Autodesk Inventor part; units mm, degrees
ref_plane "Work Plane1" through (0, 0, 0) normal (1, 0, 0) x (0, 0, -1)
ref_plane "Work Plane2" through (-0.85, -1.65, 0) normal (0, 0, 1) x (1, 0, 0)
ref_plane "Work Plane3" through (-0.85, -1.65, 0) normal (0, 0, 1) x (1, 0, 0)
ref_plane "Work Plane1" through (0, 0, 0) normal (1, 0, 0) x (0, 0, -1)
sketch "Sketch3" plane through (0, 0, 0) normal (1, 0, 0) x (0, 0, -1)
  circle A0 centre (-2.6765, 0) radius 4.3638
  line L0 (-7.0404, 0) -> (1.6873, 0)
  line L1 (-0.0184, 0) -> (-0.0184, 3.4608)
  point P0 (0, 0)
ref_plane "Work Plane2" through (-0.85, -1.65, 0) normal (0, 0, 1) x (1, 0, 0)
sketch "Sketch5" plane through (-0.85, -1.65, 0) normal (0, 0, 1) x (1, 0, 0)
  line L0 (-0.8, 2.5) -> (0, 3.3)
  line L1 (-0.8, 0.8) -> (-0.8, 2.5)
  line L2 (0, 0) -> (-0.8, 0.8)
  line L3 (2.5, 0) -> (0, 0)
  line L4 (2.5, 3.3) -> (2.5, 0)
  line L5 (0, 3.3) -> (2.5, 3.3)
  circle A0 centre (0.85, 1.65) radius 1.25
revolve "Revolution2" add sketch "Sketch3" angle 360 about axis through (0, 0, 7.0404) along (0, 0, -1) picked at (-4.6554, 0.3561) contours L1 L0 A0
ref_plane "Work Plane3" through (-0.85, -1.65, 0) normal (0, 0, 1) x (1, 0, 0)
sketch "Sketch6" plane through (-0.85, -1.65, 0) normal (0, 0, 1) x (1, 0, 0)
  line L0 (0.85, 8.4832) -> (0.85, -5.1832)
  line L1 (-0.8, 2.5) -> (0, 3.3)
  line L2 (-0.8, 0.8) -> (-0.8, 2.5)
  line L3 (0, 0) -> (-0.8, 0.8)
  line L4 (2.5, 0) -> (0, 0)
  line L5 (2.5, 3.3) -> (2.5, 0)
  line L6 (0, 3.3) -> (2.5, 3.3)
  circle A0 centre (0.85, 1.65) radius 1.25
  circle A1 centre (0.85, 1.65) radius 1.25
extrude "Extrusion2" cut sketch "Sketch6" along normal blind 2.5
properties part number "JS5210_hat_top_1"
Verification items for the finished model (mm, model axes). Coordinates: 2 decimals unless noted, no trailing zeros. Write each loop counter-clockwise with the first axis right and the second up, starting at its lowest first coordinate (ties: lowest second). Pieces come first, ordered by that corner, then holes. Notation, with made-up numbers: (17.5, 64) - (41.5, 64) arc R16 cw to (41.5, 72) - close; hole circle Ø11 at (-39.75, 87.25). An arc over 180 degrees is marked (long way). One line per question, with ' | ' between items. Start each with the question number.
1. Material ranges on line 1 along X through (y, z) = (-1.5, 2.25); line 2 along X through (y, z) = (3.25, 5); line 3 along Z through (x, y) = (1.25, 2.75), recorded low to high.
2. Gauge pin test, flat ends, axial feed: P1, Ø1.4, axis at y = -0.5, z = 1.5, coming from the +X side; P2, Ø1, axis at x = 1, y = 0, coming from the -Z side; P3, Ø2, axis at x = -2.5, z = 2.5, coming from the +Y side. Record the tip position at first contact, or that the pin passes through.
3. Draft check along Y on faces 1 (the flat face through (-1.65, 0, 1)), 2 (the flat face through (-1.5, 1.5, 0.018)). Enter one of: released by +Y, released by -Y, zero draft, split by the parting line, or undercut.
4. Section check B-B (x = -1.5). Enter the section's corners in (y, z).
5. Section check C-C (y = -0.5). Enter the section's corners in (x, z).
6. Section check A-A (z = 0.75). Enter the section's corners in (x, y).
7. Section check D-D (z = 2). Enter the section's corners in (x, y).
Computed values:
1) line 1: -4.08 to -1, 1.65 to 4.08 | line 2: -1.76 to 1.76 | line 3: 0.02 to 5.83
2) P1: x = 4.33 | P2: z = 2.5 | P3: y = 4.1
3) face 1: undercut | face 2: zero draft
4) outline: (-3.12, 0.02) - (-1, 0.02) - (-1, 2.5) - (1, 2.5) - (1, 0.02) - (3.12, 0.02) arc R4.1 ccw (long way) to start
5) outline: (-3.42, 0.02) - (-1.65, 0.02) - (-1.65, 2.5) - (1.65, 2.5) - (1.65, 0.02) - (3.42, 0.02) arc R4.34 ccw (long way) to start
6) outline: circle Ø7.83 at (0, 0); hole (-1.65, -0.85) - (-0.85, -1.65) - (1.65, -1.65) - (1.65, 1.65) - (-0.85, 1.65) - (-1.65, 0.85) - close
7) outline: circle Ø8.62 at (0, 0); hole (-1.65, -0.85) - (-0.85, -1.65) - (1.65, -1.65) - (1.65, 1.65) - (-0.85, 1.65) - (-1.65, 0.85) - close
